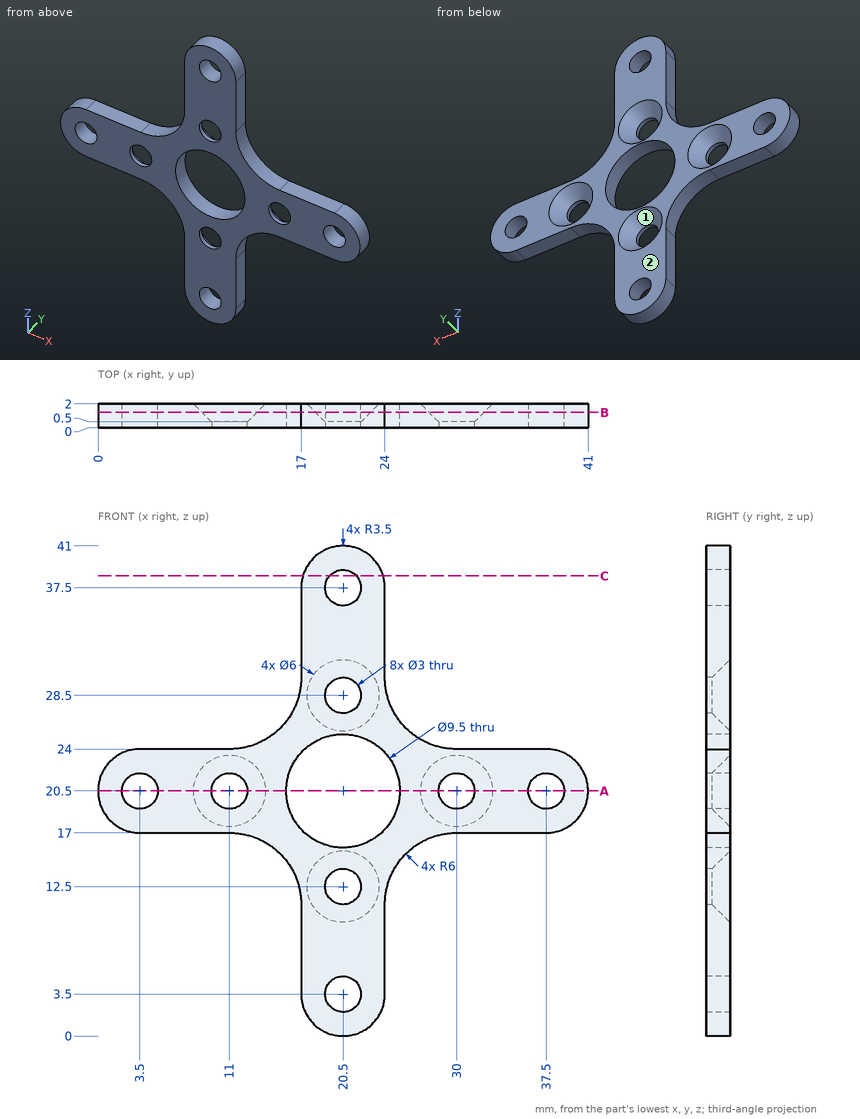
Design review of the part shown in the three views and the two pictorial views. Dimensions are in mm from the part's minimum x, y and z. Coordinates: 2 decimals unless noted, no trailing zeros. Loops run counter-clockwise (first coordinate to the right, second up) from the corner with the lowest first, then second, coordinate; pieces in that order, holes last. Notation, with made-up numbers: (-22.5, 88.5) - (25.5, 88.5) arc R16 cw to (25.5, 104.5) - close; hole circle Ø6 at (-25, -10.5). An arc over 180 degrees is marked (long way). Use a Markdown table: item, result. Add a question column.
Item 1: We need section C-C (z = 38.5). Give the boundary of the cut face in (x, y), and give its area (3 significant figures).
Item 2: For line 1 (X direction, y = 0.2, z = 20.5); line 2 (X direction, y = 1.6, z = 3.5), list the stretches that pass through material, from the lowest coordinate up.
Item 3: Insertion check: pin 1 Ø5 at (x, z) = (20.5, 3.5) entering from -Y; pin 2 Ø6 at (x, z) = (9.5, 28.5) entering from -Y; pin 3 Ø0.6 at (y, z) = (1, 7) entering from +X; pin 4 Ø0.6 at (x, y) = (8, 1) entering from -Z. Each pin has a flat end and moves straight along its axis. Give the tip position at first contact, or say it passes through.
Item 4: Mouldability with a two-part tool opening along X and no side actions: class the marked faces 1 and 2 as pulls with the +X half, pulls with the -X half, needs draft (parallel to the pull), parting line crosses it, or undercut.
Item 5: We need section B-B (y = 1.3). Give the number of separate pieces and of enclosed holes in the cut face, and give its area (3 significant figures).
Item 6: We need section A-A (z = 20.5). Give the boundary of the cut face in (x, y), and give its area (3 significant figures).
Results list:
| question | item | result |
|---|---|---|
| 1 | outline | (17.15, 0) - (19.38, 0) - (19.38, 2) - (17.15, 2) - close; (21.62, 0) - (23.85, 0) - (23.85, 2) - (21.62, 2) - close |
| 1 | area | 8.94 mm^2 |
| 2 | line 1 | x = 0 to 2, 5 to 9.5, 12.5 to 15.75, 25.25 to 28.5, 31.5 to 36, 39 to 41 |
| 2 | line 2 | x = 17 to 19, 22 to 24 |
| 3 | pin 1 | stops at y = 0 |
| 3 | pin 2 | passes through |
| 3 | pin 3 | stops at x = 24 |
| 3 | pin 4 | stops at z = 17 |
| 4 | face 1 | undercut |
| 4 | face 2 | needs draft |
| 5 | separate pieces | 1 |
| 5 | enclosed holes | 9 |
| 5 | area | 369 mm^2 |
| 6 | outline | (0, 0) - (2, 0) - (2, 2) - (0, 2) - close; (5, 0) - (9.5, 0) - (9.5, 0.5) - (8, 2) - (5, 2) - close; (12.5, 0) - (15.75, 0) - (15.75, 2) - (14, 2) - (12.5, 0.5) - close; (25.25, 0) - (28.5, 0) - (28.5, 0.5) - (27, 2) - (25.25, 2) - close; (31.5, 0) - (36, 0) - (36, 2) - (33, 2) - (31.5, 0.5) - close; (39, 0) - (41, 0) - (41, 2) - (39, 2) - close |
| 6 | area | 34.5 mm^2 |
